Geometry check sheet. Reference: the model listing, model coordinates, mm. Round coordinates to 2 decimals unless told otherwise and drop trailing zeros. Order: outer loops, then holes, each group sorted by start corner. A loop starts at its lowest first (then second) coordinate and runs counter-clockwise, first axis right, second up.
Autodesk Inventor part; units mm, degrees
ref_plane "YZ Plane" through (0, 0, 0) normal (1, 0, 0) x (0, 1, 0)
ref_plane "XZ Plane" through (0, 0, 0) normal (0, 1, 0) x (-1, 0, 0)
ref_plane "XY Plane" through (0, 0, 0) normal (0, 0, 1) x (1, 0, 0)
sketch "Sketch1" plane through (0, 0, 0) normal (1, 0, 0) x (0, 1, 0)
  line L0 (0, -277.9865) -> (0, 46.3311) construction
  line L1 (36.388, -206.3665) -> (0, 0) construction
  arc A0 (16.1301, -210.3068) -> (50.1142, -221.7774) centre (36.388, -206.3665) ccw
  line L2 (60.8363, -134.6616) -> (44.7346, -169.192) construction
  arc A1 (65.5581, -134.04) -> (58.0495, -130.7996) centre (60.8363, -134.6616) ccw
  arc A2 (72.3924, -201.9346) -> (73.9465, -197.7566) centre (69.2248, -198.3782) ccw
  arc A3 (10.1977, -165.33) -> (8.3097, -170.1013) centre (12.9846, -169.192) ccw
  line L3 (65.5581, -134.04) -> (73.9465, -197.7566)
  line L4 (72.3924, -201.9346) -> (50.1142, -221.7774)
  line L5 (16.1301, -210.3068) -> (8.3097, -170.1013)
  line L6 (69.2248, -198.3782) -> (44.7346, -169.192) construction
  line L7 (58.0495, -130.7996) -> (10.1977, -165.33)
  line L8 (44.7346, -169.192) -> (12.9846, -169.192) construction
  dimension "d8" = 209.55
  dimension "d9" = 175.006
  dimension "d11" = 10
  dimension "d12" = 20.6375
  dimension "d13" = 38.1
  dimension "d14" = 25
  dimension "d19" = 4.7625
  dimension "d37" = 40
  dimension "d39" = 90
  dimension "d40" = 31.75
  dimension "d41" = 38.1
extrude "Plate1" add sketch "Sketch1" along normal blind 3.175
hole "Hole1" at (0, 60.8363, -134.6616) at (0, 12.9846, -169.192) at (0, 69.2248, -198.3782) direction (1, 0, 0) diameter 4.9784 end through all
hole "Hole2" at (0, 36.388, -206.3665) at (0, 44.7346, -169.192) direction (1, 0, 0) diameter 28.575 end through all
sketch "Sketch2" plane through (3.175, 0, 0) normal (1, 0, 0) x (0, 0, -1)
  circle A0 centre (169.192, 44.7346) radius 14.2875
  circle A1 centre (206.3665, 36.388) radius 14.2875
  circle A2 centre (198.3782, 69.2248) radius 2.4892
  circle A3 centre (169.192, 12.9846) radius 2.4892
  circle A4 centre (134.6616, 60.8363) radius 2.4892
  arc A5 (134.04, 65.5581) -> (130.7996, 58.0495) centre (134.6616, 60.8363) ccw
  line L0 (165.33, 10.1977) -> (130.7996, 58.0495)
  arc A6 (165.33, 10.1977) -> (170.1013, 8.3097) centre (169.192, 12.9846) ccw
  line L1 (210.3068, 16.1301) -> (170.1013, 8.3097)
  arc A7 (210.3068, 16.1301) -> (221.7774, 50.1142) centre (206.3665, 36.388) ccw
  line L2 (201.9346, 72.3924) -> (221.7774, 50.1142)
  arc A8 (201.9346, 72.3924) -> (197.7566, 73.9465) centre (198.3782, 69.2248) ccw
  line L3 (134.04, 65.5581) -> (197.7566, 73.9465)
  line L4 (134.6616, 60.8363) -> (198.3782, 69.2248)
  line L5 (198.3782, 69.2248) -> (218.221, 46.9466)
  arc A9 (209.3975, 20.805) -> (218.221, 46.9466) centre (206.3665, 36.388) ccw
  line L6 (209.3975, 20.805) -> (169.192, 12.9846)
  line L7 (169.192, 12.9846) -> (134.6616, 60.8363)
  circle A10 centre (134.6616, 60.8363) radius 4.7625
  circle A11 centre (198.3782, 69.2248) radius 4.7625
  circle A12 centre (169.192, 12.9846) radius 4.7625
  circle A13 centre (169.192, 44.7346) radius 22.225
  circle A14 centre (206.3665, 36.388) radius 20.6375
  point P0 (0, 0)
  point P1 (196.4534, 18.2872)
  point P2 (186.5015, 30.7943)
  point P3 (161.2634, 23.9719)
  point P4 (166.4051, 16.8466)
  point P5 (173.8668, 13.8939)
  point P6 (190.7995, 49.937)
  point P7 (209.4503, 56.7938)
  point P8 (201.5458, 65.6684)
  point P9 (193.6565, 68.6032)
  point P10 (175.0995, 66.1601)
  point P11 (146.9886, 43.7537)
  point P12 (157.9404, 63.901)
  point P13 (139.3834, 61.458)
  point P14 (137.4485, 56.9744)
  dimension "d42" = 4.7625
  dimension "d44" = 41.275
  dimension "d45" = 44.45
extrude "Cut1" cut sketch "Sketch2" against normal blind 3.175 contours A11 L5 A14 A13 L4 | A13 L7 A10 L4 | A14 L6 A12 L7 A13
fillet "Corner Round1" radius 1.5875 14 edges at (1.5875, 43.7537, -146.9886) (1.5875, 63.901, -157.9404) (1.5875, 56.9744, -137.4485) (1.5875, 56.7938, -209.4503) (1.5875, 30.7943, -186.5015) (1.5875, 13.8939, -173.8668) (1.5875, 18.2872, -196.4534) (1.5875, 49.937, -190.7995) (1.5875, 61.458, -139.3834) (1.5875, 68.6032, -193.6565) (1.5875, 65.6684, -201.5458) (1.5875, 66.1601, -175.0995) (1.5875, 16.8466, -166.4051) (1.5875, 23.9719, -161.2634)
equation "\"d25\" = Thickness"
equation "\"d46\" = Thickness"
equation "\"d7\" = Thickness"
equation "\"BendRadius\" = Thickness"
equation "\"BendReliefWidth\" = Thickness"
equation "\"BendReliefDepth\" = 0.5 * Thickness"
equation "\"CornerReliefSize\" = 4 * Thickness"
equation "\"MinimumRemnant\" = 2 * Thickness"
equation "\"TransitionRadius\" = BendRadius"
equation "\"JacobiRadiusSize\" = BendRadius"
equation "\"GapSize\" = Thickness"
properties part number "PLATE,BEARING,MOUNT"
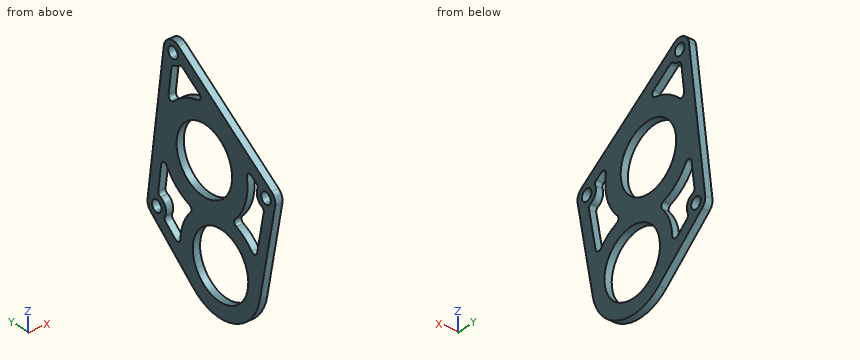
(1) Material ranges on line 1 (Z direction, x = 1.85, y = 34); line 2 (Y direction, x = 0.7, z = -171); line 3 (Z direction, x = 2.55, y = 51), recorded low to high.
Returned:
line 1: z = -226.87 to -220.45, -192.28 to -178.62, -159.76 to -148.15
line 2: y = 8.48 to 11.27, 14.7 to 17.39, 22.58 to 30.56, 58.91 to 70.42
line 3: z = -220.99 to -182.03, -156.35 to -147.87, -141.76 to -135.89
(2) Sectioned sample at D-D, the plane x = 2.5. Give the number of separate pieces and of enclosed holes in the cut face, and give its area (3 significant figures).
Returned:
separate pieces: 1
enclosed holes: 8
area: 2,380 mm2
(3) Sectioned sample at B-B, the plane z = -214.5. Record the cut outline in (x, y) (3 decimals), and give its area (3 significant figures).
Returned:
outline: (0, 17.421) - (3.175, 17.421) - (3.175, 24.642) - (0, 24.642) - close; (0, 48.134) - (3.175, 48.134) - (3.175, 58.285) - (0, 58.285) - close
area: 55.2 mm2
(4) Sectioned sample at C-C, the plane y = 34. Record the cut outline in (x, z) (3 decimals).
Returned:
outline: (0, -226.865) - (3.175, -226.865) - (3.175, -220.453) - (0, -220.453) - close; (0, -192.28) - (3.175, -192.28) - (3.175, -178.621) - (0, -178.621) - close; (0, -159.763) - (3.175, -159.763) - (3.175, -148.154) - (0, -148.154) - close
(5) Sectioned sample at A-A, the plane z = -204. Record the cut outline in (x, y) (1 decimal), and give its area (3 significant figures).
Returned:
outline: (0, 14.9) - (3.2, 14.9) - (3.2, 22.3) - (0, 22.3) - close; (0, 50.5) - (3.2, 50.5) - (3.2, 56.9) - (0, 56.9) - close; (0, 62.9) - (3.2, 62.9) - (3.2, 70.1) - (0, 70.1) - close
area: 66.6 mm2
(6) Depth check by flat-ended pin: P1, Ø1.5, axis at x = 1, y = 64, coming from the -Z side. Enter the tip coordinate at first touch or a pass-through.
Returned:
P1: stops at z = -210.08
